Verification items for the finished model (mm, model axes). Face numbers are marked on the shaded views. A direction names the side the tool comes from. Round coordinates to 2 decimals unless told otherwise and drop trailing zeros. Order: outer loops, then holes, each group sorted by start corner. A loop starts at its lowest first (then second) coordinate and runs counter-clockwise, first axis right, second up. Notation, with made-up numbers: (0, 86.25) -> (46, 86.25) arc R10 ccw to (46, 99.25) -> close; hole circle Ø10 at (75, 28). An arc over 180 degrees is marked (long way). Put each result on its own line as item: value.
from build123d import *

# Parameters (mm, degrees)
BOSS_EXTRUDE1_DEPTH = 12
SKETCH2_R           = 2.5
CUT_EXTRUDE1_DEPTH  = 500
SKETCH4_W           = 35
SKETCH4_H           = 50
BOSS_EXTRUDE2_DEPTH = 30
BOSS_EXTRUDE3_DEPTH = 35
FILLET1_R           = 5
FILLET2_R           = 1
FILLET_1_R          = 1


with BuildPart() as part:
    # Sketch1 → Boss-Extrude1 (new body)
    with BuildSketch(Plane(origin=(0, 0, 0), x_dir=(1, 0, 0), z_dir=(0, 1, 0))):
        with BuildLine():
            Line((-41.057019736, 28.536312488), (-53.951781887, 28.536312488))
            ThreePointArc((-53.951781887, 28.536312488), (-55.779259556, -24.774787639), (-15, -59.16177735))
            Line((-15, -59.16177735), (15, -59.16177735))
            ThreePointArc((15, -59.16177735), (55.779259556, -24.774787639), (53.951781887, 28.536312488))
            Line((53.951781887, 28.536312488), (41.057019736, 28.536312488))
            ThreePointArc((41.057019736, 28.536312488), (0, -50), (-41.057019736, 28.536312488))
        make_face()
        with BuildLine():
            ThreePointArc((15, -59.16177735), (0, -61.033727554), (-15, -59.16177735))
            Line((-15, -59.16177735), (-15, -124.16177735))
            Line((-15, -124.16177735), (15, -124.16177735))
            Line((15, -124.16177735), (15, -59.16177735))
        make_face()
        with BuildLine():
            Line((15, -59.16177735), (-15, -59.16177735))
            ThreePointArc((-15, -59.16177735), (0, -61.033727554), (15, -59.16177735))
        make_face()
    extrude(amount=BOSS_EXTRUDE1_DEPTH)

    # Sketch2 → Cut-Extrude1 (cut, symmetric)
    with BuildSketch(Plane(origin=(15, 0, 0), x_dir=(0, 0, -1), z_dir=(1, 0, 0))):
        with Locations((0, 6)):
            Circle(SKETCH2_R)
    extrude(amount=CUT_EXTRUDE1_DEPTH, both=True, mode=Mode.SUBTRACT)

    # Sketch4 → Boss-Extrude2 (add)
    with BuildSketch(Plane.ZY.offset(15)):
        with Locations((106.66177735, 37)):
            Rectangle(SKETCH4_W, SKETCH4_H)
    extrude(amount=-BOSS_EXTRUDE2_DEPTH)

    # Sketch5 → Boss-Extrude3 (add)
    with BuildSketch(Plane.XY.offset(124.16177735)):
        with BuildLine():
            Line((-11.643875535, 94.635635732), (-14.586391276, 94.635635732))
            ThreePointArc((-14.586391276, 94.635635732), (-17.06618452, 88.984526001), (-17.437258677, 82.824435117))
            Line((-17.437258677, 82.824435117), (-15, 62))
            Line((-15, 62), (15, 62))
            Line((15, 62), (17.437258677, 82.824435117))
            ThreePointArc((17.437258677, 82.824435117), (17.06618452, 88.984526001), (14.586391276, 94.635635732))
            Line((14.586391276, 94.635635732), (11.643875535, 94.635635732))
            ThreePointArc((11.643875535, 94.635635732), (0, 69.665264065), (-11.643875535, 94.635635732))
        make_face()
    extrude(amount=-BOSS_EXTRUDE3_DEPTH)

    # Fillet1
    fillet1_edges = [part.edges().sort_by_distance(p)[0] for p in [
        (-53.951781887, 6, -28.536312488),
        (-41.057019736, 6, -28.536312488),
        (41.057019736, 6, -28.536312488),
        (53.951781887, 6, -28.536312488),
    ]]
    fillet(fillet1_edges, radius=FILLET1_R)

    # Fillet2
    fillet2_edges = [part.edges().sort_by_distance(p)[0] for p in [
        (11.643875535, 94.635635732, 106.66177735),
        (-11.643875535, 94.635635732, 106.66177735),
    ]]
    fillet(fillet2_edges, radius=FILLET2_R)

    # 圆角1
    fillet_1_edges = [part.edges().sort_by_distance(p)[0] for p in [
        (14.586391276, 94.635635732, 106.66177735),
        (-14.586391276, 94.635635732, 106.66177735),
    ]]
    fillet(fillet_1_edges, radius=FILLET_1_R)


solid = part.part
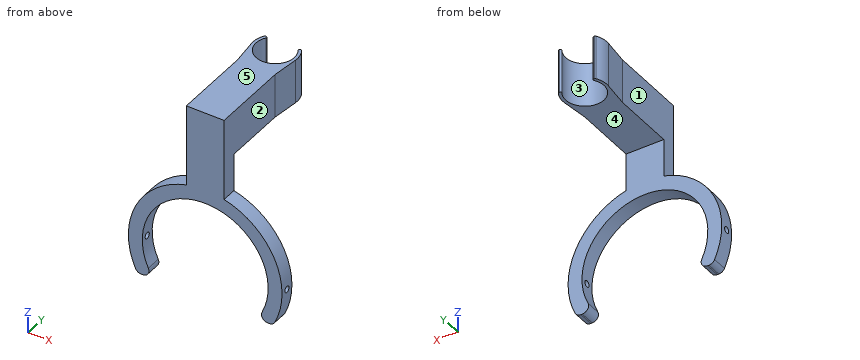
Item 1: Section check C-C on y = 6. Record the boundary of the cut face in (x, z), then the cut area to 3 significant figures.
Check sheet entries:
outline: (-60.98, -2.5) arc R61.03 ccw to (-55.39, -25.64) arc R5 ccw to (-50.85, -28.54) -> (-49.71, -28.54) arc R5 ccw to (-45.19, -21.4) arc R50 cw to (-49.94, -2.5) -> close; (-60.98, 2.5) -> (-49.94, 2.5) arc R50 cw to (49.94, 2.5) -> (60.98, 2.5) arc R61.03 ccw to (15, 59.16) -> (15, 124.16) -> (-15, 124.16) -> (-15, 59.16) arc R61.03 ccw to start; (45.19, -21.4) arc R5 ccw to (49.71, -28.54) -> (50.85, -28.54) arc R5 ccw to (55.39, -25.64) arc R61.03 ccw to (60.98, -2.5) -> (49.94, -2.5) arc R50 cw to start
area: 4,350 mm^2
Item 2: Section check A-A on z = 0. Record the boundary of the cut face in (x, y), then the cut area to 3 significant figures.
Check sheet entries:
outline: (-61.03, 0) -> (-50, 0) -> (-50, 3.5) -> (-61.03, 3.5) -> close; (-61.03, 8.5) -> (-50, 8.5) -> (-50, 12) -> (-61.03, 12) -> close; (50, 0) -> (61.03, 0) -> (61.03, 3.5) -> (50, 3.5) -> close; (50, 8.5) -> (61.03, 8.5) -> (61.03, 12) -> (50, 12) -> close
area: 154 mm^2
Item 3: Section check D-D on x = 0. Record the boundary of the cut face in (y, z).
Check sheet entries:
outline: (0, 50) -> (12, 50) -> (12, 89.16) -> (69.67, 89.16) -> (69.67, 124.16) -> (0, 124.16) -> close
Item 4: Gauge pin test, flat ends, axial feed: pin 1 Ø18.5 at (y, z) = (33.5, 94) entering from -X; pin 2 Ø10.5 at (x, y) = (7, 38.5) entering from -Z. Record the tip position at first contact, or that the pin passes through.
Check sheet entries:
pin 1: stops at x = -15
pin 2: stops at z = 89.16
Item 5: Release check for a two-part mould opening along X. For the marked faces 1, 2 and 3 record: +X half, -X half, draft (parallel to the pull), parting line (faces both ways), or undercut.
Check sheet entries:
face 1: -X half
face 2: +X half
face 3: undercut
Item 6: Tool access check on the marked faces 4 and 5. Record the directions out of +Z, -Z, +X, -X, +Y, -Y that give a thin tool (end or side, any length) a straight path to the whole face; none if there is none.
Check sheet entries:
face 4: -Z, +X, -X, +Y
face 5: +Z, +X, -X, +Y, -Y
Item 7: Section check B-B on x = -47. Record the boundary of the cut face in (y, z), then the cut area to 3 significant figures.
Check sheet entries:
outline: (0, -27.74) -> (12, -27.74) -> (12, -17.06) -> (0, -17.06) -> close; (0, 17.06) -> (12, 17.06) -> (12, 38.94) -> (0, 38.94) -> close
area: 391 mm^2
Item 8: Material ranges on L1, parallel to Y at x = -52.25, z = 0; L2, parallel to X at y = 2, z = 0; L3, parallel to Z at x = 15, y = 82, recorded low to high. Write a range as [from, to].
Check sheet entries:
L1: y = [0, 3.5], [8.5, 12]
L2: x = [-61.03, -50], [50, 61.03]
L3: z = [89.16, 124.16]
